```python
from build123d import *

# Parameters (mm, degrees)
SKETCH1_W           = 20
SKETCH1_H           = 13.42
BOSS_EXTRUDE1_DEPTH = 10.33
SKETCH2_R           = 1.25
CUT_EXTRUDE1_DEPTH  = 10.33


with BuildPart() as part:
    # Sketch1 → Boss-Extrude1 (new body)
    with BuildSketch(Plane.YZ):
        Rectangle(SKETCH1_W, SKETCH1_H)
    extrude(amount=BOSS_EXTRUDE1_DEPTH)

    # Sketch2 → Cut-Extrude1 (cut)
    with BuildSketch(Plane(origin=(10.33, 0, 0), x_dir=(0, 0, -1), z_dir=(1, 0, 0))):
        with Locations((0, 5)):
            Circle(SKETCH2_R)
        with Locations((0, -5)):
            Circle(SKETCH2_R)
    extrude(amount=-CUT_EXTRUDE1_DEPTH, mode=Mode.SUBTRACT)


solid = part.part
```
Verification items for the finished model (mm, model axes). Give positions to 0.01 mm unless a question says otherwise; leave off trailing zeros. Order: outer loops, then holes, each group sorted by start corner. A loop starts at its lowest first (then second) coordinate and runs counter-clockwise, first axis right, second up. Notation, with made-up numbers: M 81.5,29.25 L 105.5,29.25 A16 ccw 105.5,56.25 Z; hole C 32.5,25.5 d2. An arc over 180 degrees is marked long. Return JSON: item names as keys, results as strings. Group by question number.
1) Section check B-B on z = 0. Record the cut outline in (x, y).
2) Section check A-A on y = 5. Record the cut outline in (x, z), and give its area (3 significant figures).
3) Mould release check, pull along Z, two halves, no side actions. Record for faces 1 (the face through (5, 0, -6.71)), 2 (the face through (5.24, 3.78, 0.27)), 3 (the face through (5, -10, 0)): pulls with the +Z half, pulls with the -Z half, needs draft (parallel to the pull), parting line crosses it, or undercut.
4) Scan lines: line 1 (Y direction, x = 6.5, z = 0); line 2 (Z direction, x = 5.5, y = -4.5). Record each from-to range of solid material in increasing order.
5) Section check C-C on x = 6.25. Record the cut outline in (y, z), and give its area (3 significant figures).
6) Go/stop test with a flat-tipped pin: pin 1 Ø3 at (y, z) = (5, 0) entering from +X. Record where the tip stops, or that it passes through.
Answer block:
{
 "1": {"outline": "M 0,-10 L 10.33,-10 L 10.33,-6.25 L 0,-6.25 Z; M 0,-3.75 L 10.33,-3.75 L 10.33,3.75 L 0,3.75 Z; M 0,6.25 L 10.33,6.25 L 10.33,10 L 0,10 Z"},
 "2": {"outline": "M 0,-6.71 L 10.33,-6.71 L 10.33,-1.25 L 0,-1.25 Z; M 0,1.25 L 10.33,1.25 L 10.33,6.71 L 0,6.71 Z", "area": "113 mm^2"},
 "3": {"face 1": "pulls with the -Z half", "face 2": "undercut", "face 3": "needs draft"},
 "4": {"line 1": "y = -10 to -6.25, -3.75 to 3.75, 6.25 to 10", "line 2": "z = -6.71 to -1.15, 1.15 to 6.71"},
 "5": {"outline": "M -10,-6.71 L 10,-6.71 L 10,6.71 L -10,6.71 Z; hole C -5,0 d2.5; hole C 5,0 d2.5", "area": "259 mm^2"},
 "6": {"pin 1": "stops at x = 10.33"}
}
